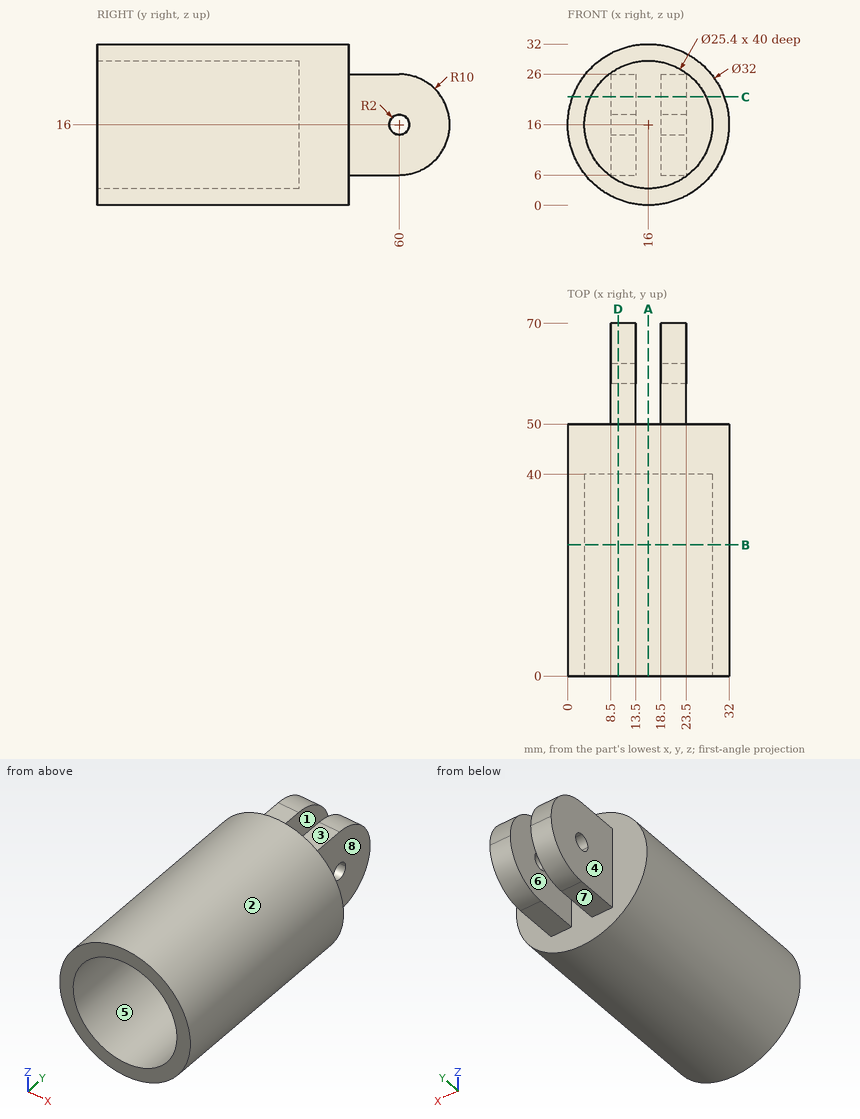
Geometry check sheet. Reference: drawing and pictorial views, mm from the part's lowest x, y, z. A direction names the side the tool comes from. Round coordinates to 2 decimals unless told otherwise and drop trailing zeros. Loops run counter-clockwise (first coordinate to the right, second up) from the corner with the lowest first, then second, coordinate; pieces in that order, holes last. Notation, with made-up numbers: (42.5, -9) - (70.5, -9) arc R28 cw to (70.5, 24) - close; hole circle Ø10 at (33, 9). An arc over 180 degrees is marked (long way). Answer in a Markdown table with one row per item. Add a question column.
Q1. Section check B-B on y = 26. Enter the section's corners in (x, z).
Q2. Material ranges on line 1 (X direction, y = 60, z = 7); line 2 (Z direction, x = 15.5, y = 29.5); line 3 (X direction, y = 11, z = 16), recorded low to high.
Q3. Gauge pin test, flat ends, axial feed: pin 1 (2.5 mm diameter, centred on x = 10.5, y = 57.5, fed in from +Z); pin 2 (4 mm diameter, centred on x = 27.5, y = 46.5, fed in from +Z); pin 3 (4 mm diameter, centred on x = 12, y = 53.5, fed in from -Z). Record the tip position at first contact, or that the pin passes through.
Q4. Section check C-C on z = 21.5. Enter the section's corners in (x, y), plus the area to 3 significant figures.
Q5. Section check D-D on x = 10. Enter the section's corners in (y, z).
Q6. Tool access check on the marked faces 4, 5, 6, 7 and 8. Record the directions out of +Z, -Z, +X, -X, +Y, -Y that give a thin tool (end or side, any length) a straight path to the whole face; none if there is none.
Q7. Section check A-A on x = 16. Enter the section's corners in (y, z), plus the area to 3 significant figures.
Q8. Release check for a two-part mould opening along X. For the marked faces 1, 2 and 3 record: pulls with the +X half, pulls with the -X half, needs draft (parallel to the pull), parting line crosses it, or undercut.
Found:
| question | item | result |
|---|---|---|
| 1 | outline | circle Ø32 at (16, 16); hole circle Ø25.4 at (16, 16) |
| 2 | line 1 | x = 8.5 to 13.5, 18.5 to 23.5 |
| 2 | line 2 | z = 0.01 to 3.31, 28.69 to 31.99 |
| 2 | line 3 | x = 0 to 3.3, 28.7 to 32 |
| 3 | pin 1 | stops at z = 26 |
| 3 | pin 2 | stops at z = 28.87 |
| 3 | pin 3 | stops at z = 6 |
| 4 | outline | (0.98, 0) - (4.55, 0) - (4.55, 40) - (27.45, 40) - (27.45, 0) - (31.02, 0) - (31.02, 50) - (23.5, 50) - (23.5, 68.35) - (18.5, 68.35) - (18.5, 50) - (13.5, 50) - (13.5, 68.35) - (8.5, 68.35) - (8.5, 50) - (0.98, 50) - close |
| 4 | area | 770 mm² |
| 5 | outline | (0, 1.17) - (50, 1.17) - (50, 6) - (60, 6) arc R10 ccw to (60, 26) - (50, 26) - (50, 30.83) - (0, 30.83) - (0, 27.19) - (40, 27.19) - (40, 4.81) - (0, 4.81) - close; hole circle Ø4 at (60, 16) |
| 6 | face 4 | +Z, -Z, -X, +Y |
| 6 | face 5 | -Y |
| 6 | face 6 | +Z, -Z, +Y |
| 6 | face 7 | -Z, +X, -X, +Y |
| 6 | face 8 | +Z, -Z, +X, +Y |
| 7 | outline | (0, 0) - (50, 0) - (50, 32) - (0, 32) - (0, 28.7) - (40, 28.7) - (40, 3.3) - (0, 3.3) - close |
| 7 | area | 584 mm² |
| 8 | face 1 | undercut |
| 8 | face 2 | parting line crosses it |
| 8 | face 3 | needs draft |
